Read the model definition and answer for the solid it produces. Units are mm, in the model's axes. A direction names the side the tool comes from. Round coordinates to 2 decimals unless told otherwise and drop trailing zeros. Order: outer loops, then holes, each group sorted by start corner. A loop starts at its lowest first (then second) coordinate and runs counter-clockwise, first axis right, second up.
from build123d import *

# Parameters (mm, degrees)
CROQUIS1_W              = 64
CROQUIS1_H              = 64
SALIENTE_EXTRUIR1_DEPTH = 60
CROQUIS2_W              = 70
CROQUIS2_H              = 70
CROQUIS2_W_2            = 64
CROQUIS2_H_2            = 64
SALIENTE_EXTRUIR2_DEPTH = 64
CORTAR_EXTRUIR1_DEPTH   = 21
CROQUIS5_R              = 1.1
CORTAR_EXTRUIR2_DEPTH   = 10
CORTAR_EXTRUIR3_REACH   = 30
CROQUIS10_R             = 4.5
CROQUIS11_W             = 70
CROQUIS11_H             = 70
CORTAR_EXTRUIR4_DEPTH   = 30
CROQUIS12_W             = 23
CROQUIS12_H             = 12.2
CORTAR_EXTRUIR5_DEPTH   = 21
CORTAR_EXTRUIR6_REACH   = 30
CROQUIS13_R             = 4.5
CROQUIS14_R             = 1.1
CORTAR_EXTRUIR7_DEPTH   = 10
CROQUIS15_R             = 3.7
CORTAR_EXTRUIR8_DEPTH   = 10
CROQUIS16_W             = 64
CROQUIS16_H             = 64
CORTAR_EXTRUIR9_DEPTH   = 5
CROQUIS17_W             = 12.5
CROQUIS17_H             = 12.998685397
CORTAR_EXTRUIR10_DEPTH  = 5
CORTAR_EXTRUIR11_REACH  = 72
CROQUIS18_W             = 70
CROQUIS18_H             = 9
CROQUIS18_H_2           = 5.000169364
CORTAR_EXTRUIR13_DEPTH  = 5
CORTAR_EXTRUIR14_REACH  = 12
CROQUIS21_W             = 81.467019472
CROQUIS21_H             = 81.467019472
CORTAR_EXTRUIR16_REACH  = 5.001
CROQUIS23_W             = 3.1
CROQUIS23_H             = 12.5


with BuildPart() as part:
    # Croquis1 → Saliente-Extruir1 (new body)
    with BuildSketch(Plane(origin=(0, 0, 0), x_dir=(1, 0, 0), z_dir=(0, 1, 0))):
        Rectangle(CROQUIS1_W, CROQUIS1_H)
    extrude(amount=SALIENTE_EXTRUIR1_DEPTH)

    # Croquis2 → Saliente-Extruir2 (add)
    with BuildSketch(Plane(origin=(0, 0, 0), x_dir=(1, 0, 0), z_dir=(0, 1, 0))):
        Rectangle(CROQUIS2_W, CROQUIS2_H)
        Rectangle(CROQUIS2_W_2, CROQUIS2_H_2, mode=Mode.SUBTRACT)
    extrude(amount=SALIENTE_EXTRUIR2_DEPTH)

    # Croquis4 → Cortar-Extruir1 (cut)
    with BuildSketch(Plane(origin=(0, 60, 0), x_dir=(1, 0, 0), z_dir=(0, 1, 0))):
        Polygon((-7, 6), (-7, -6), (-7, -6.25), (16, -6.25), (16, -6), (16, 6), (16, 6.25), (-7, 6.25), align=None)
    extrude(amount=-CORTAR_EXTRUIR1_DEPTH, mode=Mode.SUBTRACT)

    # Croquis5 → Cortar-Extruir2 (cut)
    with BuildSketch(Plane(origin=(0, 60, 0), x_dir=(1, 0, 0), z_dir=(0, 1, 0))):
        with Locations((19, 0)):
            Circle(CROQUIS5_R)
        with Locations((-9, 0)):
            Circle(CROQUIS5_R)
    extrude(amount=-CORTAR_EXTRUIR2_DEPTH, mode=Mode.SUBTRACT)

    # Croquis10 → Cortar-Extruir3 (cut, up to next)
    with BuildSketch(Plane(origin=(-7, 0, 0), x_dir=(0, 0, -1), z_dir=(1, 0, 0)), mode=Mode.PRIVATE) as cortar_extruir3_sk1:
        with Locations((0, 44)):
            Circle(CROQUIS10_R)
    cortar_extruir3_tool1 = extrude(cortar_extruir3_sk1.sketch, amount=-CORTAR_EXTRUIR3_REACH, mode=Mode.PRIVATE) & part.part
    add(cortar_extruir3_tool1.solids().sort_by_distance((-7, 44, 0))[0], mode=Mode.SUBTRACT)

    # Croquis11 → Cortar-Extruir4 (cut)
    with BuildSketch(Plane.XZ):
        Rectangle(CROQUIS11_W, CROQUIS11_H)
    extrude(amount=-CORTAR_EXTRUIR4_DEPTH, mode=Mode.SUBTRACT)

    # Croquis12 → Cortar-Extruir5 (cut)
    with BuildSketch(Plane.XZ.offset(-30)):
        with Locations((4.5, 22.1)):
            Rectangle(CROQUIS12_W, CROQUIS12_H)
    extrude(amount=-CORTAR_EXTRUIR5_DEPTH, mode=Mode.SUBTRACT)

    # Croquis13 → Cortar-Extruir6 (cut, up to next)
    with BuildSketch(Plane(origin=(-7, 0, 0), x_dir=(0, 0, -1), z_dir=(1, 0, 0)), mode=Mode.PRIVATE) as cortar_extruir6_sk1:
        with Locations((-22.1, 46)):
            Circle(CROQUIS13_R)
    cortar_extruir6_tool1 = extrude(cortar_extruir6_sk1.sketch, amount=-CORTAR_EXTRUIR6_REACH, mode=Mode.PRIVATE) & part.part
    add(cortar_extruir6_tool1.solids().sort_by_distance((-7, 46, 22.1))[0], mode=Mode.SUBTRACT)

    # Croquis14 → Cortar-Extruir7 (cut)
    with BuildSketch(Plane.XZ.offset(-30)):
        with Locations((19, 22.1)):
            Circle(CROQUIS14_R)
        with Locations((-9, 22.1)):
            Circle(CROQUIS14_R)
    extrude(amount=-CORTAR_EXTRUIR7_DEPTH, mode=Mode.SUBTRACT)

    # Croquis15 → Cortar-Extruir8 (cut)
    with BuildSketch(Plane.XZ.offset(-30)):
        with Locations((0, -22.1)):
            Circle(CROQUIS15_R)
    extrude(amount=-CORTAR_EXTRUIR8_DEPTH, mode=Mode.SUBTRACT)

    # Croquis16 → Cortar-Extruir9 (cut)
    with BuildSketch(Plane(origin=(0, 60, 0), x_dir=(1, 0, 0), z_dir=(0, 1, 0))):
        Rectangle(CROQUIS16_W, CROQUIS16_H)
    extrude(amount=-CORTAR_EXTRUIR9_DEPTH, mode=Mode.SUBTRACT)

    # Croquis17 → Cortar-Extruir10 (cut)
    with BuildSketch(Plane(origin=(-7, 0, 0), x_dir=(0, 0, -1), z_dir=(1, 0, 0))):
        with Locations((0, 45.499342699)):
            Rectangle(CROQUIS17_W, CROQUIS17_H)
    extrude(amount=-CORTAR_EXTRUIR10_DEPTH, mode=Mode.SUBTRACT)

    # Croquis18 → Cortar-Extruir11 (cut, up to next)
    with BuildSketch(Plane(origin=(35, 0, 0), x_dir=(0, 0, -1), z_dir=(1, 0, 0)), mode=Mode.PRIVATE) as cortar_extruir11_sk1:
        with Locations((0, 59.5)):
            Rectangle(CROQUIS18_W, CROQUIS18_H)
    cortar_extruir11_tool1 = extrude(cortar_extruir11_sk1.sketch, amount=-CORTAR_EXTRUIR11_REACH, mode=Mode.PRIVATE) & part.part
    add(cortar_extruir11_tool1.solids().sort_by_distance((35, 59.5, 0))[0], mode=Mode.SUBTRACT)
    # Croquis18 → Cortar-Extruir11 (cut, up to next)
    with BuildSketch(Plane(origin=(35, 0, 0), x_dir=(0, 0, -1), z_dir=(1, 0, 0)), mode=Mode.PRIVATE) as cortar_extruir11_sk2:
        with Locations((0, 32.500084682)):
            Rectangle(CROQUIS18_W, CROQUIS18_H_2)
    cortar_extruir11_tool2 = extrude(cortar_extruir11_sk2.sketch, amount=-CORTAR_EXTRUIR11_REACH, mode=Mode.PRIVATE) & part.part
    add(cortar_extruir11_tool2.solids().sort_by_distance((35, 32.500085, 0))[0], mode=Mode.SUBTRACT)

    # Croquis19 → Cortar-Extruir13 (cut)
    with BuildSketch(Plane(origin=(-7, 0, 0), x_dir=(0, 0, -1), z_dir=(1, 0, 0))):
        Polygon((-16, 51), (-28.2, 51), (-28.2, 38.000169364), (-22.1, 38.000169364), (-16, 38.000169364), align=None)
    extrude(amount=-CORTAR_EXTRUIR13_DEPTH, mode=Mode.SUBTRACT)

    # Croquis21 → Cortar-Extruir14 (cut, up to next)
    with BuildSketch(Plane(origin=(0, 45.000169364, 0), x_dir=(-1, 0, 0), z_dir=(0, -1, 0)), mode=Mode.PRIVATE) as cortar_extruir14_sk1:
        with Locations((0.076423095, -0.764230952)):
            Rectangle(CROQUIS21_W, CROQUIS21_H)
    cortar_extruir14_tool1 = extrude(cortar_extruir14_sk1.sketch, amount=CORTAR_EXTRUIR14_REACH, mode=Mode.PRIVATE) & part.part
    add(cortar_extruir14_tool1.solids().sort_by_distance((-0.076423, 45.000169, 0.764231))[0], mode=Mode.SUBTRACT)

    # Croquis23 → Cortar-Extruir16 (cut, up to next)
    with BuildSketch(Plane.XZ.offset(-51.998685397), mode=Mode.PRIVATE) as cortar_extruir16_sk1:
        with Locations((-8.55, 0)):
            Rectangle(CROQUIS23_W, CROQUIS23_H)
    cortar_extruir16_tool1 = extrude(cortar_extruir16_sk1.sketch, amount=-CORTAR_EXTRUIR16_REACH, mode=Mode.PRIVATE) & part.part
    add(cortar_extruir16_tool1.solids().sort_by_distance((-8.55, 51.998685, 0))[0], mode=Mode.SUBTRACT)


solid = part.part
Q1. A cutting plane is placed at C-C, the plane y = 46. Give the vertices of the cut face in (x, z).
Outcome:
outline: (-35, -35) - (35, -35) - (35, 35) - (-35, 35) - (-35, 26.6) - (-12, 26.6) - (-12, 28.2) - (16, 28.2) - (16, 16) - (-12, 16) - (-12, 17.6) - (-35, 17.6) - (-35, 4.03) - (-12, 4.03) - (-12, 6.25) - (16, 6.25) - (16, -6.25) - (-12, -6.25) - (-12, -4.03) - (-35, -4.03) - close
Q2. A cutting plane is placed at D-D, the plane x = 19. Give the vertices of the cut face in (y, z).
Outcome:
outline: (45, -35) - (55, -35) - (55, -1.1) - (50, -1.1) - (50, 1.1) - (55, 1.1) - (55, 35) - (45, 35) - close
Q3. A cutting plane is placed at B-B, the plane z = 22.1. Give the vertices of the cut face in (x, y), plus the area to 3 significant figures.
Outcome:
outline: (-35, 50.5) - (-12, 50.5) - (-12, 51) - (16, 51) - (16, 45) - (35, 45) - (35, 55) - (-35, 55) - close
area: 405 mm2
Q4. For a pull along X with two mould halves and no side action, classify faces 1 (the face through (16, 50, 0)), 2 (the face through (2, 48, 28.2)), 3 (the face through (35, 50, 0)), 4 (the face through (0, 45, -8)) as released by +X, released by -X, zero draft, split by the parting line, or undercut.
Outcome:
face 1: undercut
face 2: undercut
face 3: released by +X
face 4: zero draft
Q5. Flat-ended cylindrical pins translate along their axes: pin 1 (10 mm diameter, centred on x = 1.5, z = 23, fed in from -Y); pin 2 (0.6 mm diameter, centred on x = -10.5, z = -2, fed in from -Y); pin 3 (2 mm diameter, centred on x = 19, z = 0, fed in from +Y). Find the tip coordinate at first contact, or state that the pin passes through.
Outcome:
pin 1: stops at y = 51
pin 2: stops at y = 52
pin 3: stops at y = 50
Q6. For faces 5 (the face through (-23.3, 50.5, 22)), 6 (the face through (-11, 51.999, 0)), 7 (the face through (17.9, 52.5, 0)), determine the directions among +Z, -Z, +X, -X, +Y, -Y from which every point of the face is accessible in a straight line to the end or side of a thin tool.
Outcome:
face 5: -X
face 6: -Y
face 7: +Y
Q7. A cutting plane is placed at A-A, the plane z = 0. Give the vertices of the cut face in (x, y).
Outcome:
outline: (-35, 48.5) - (-12, 48.5) - (-12, 52) - (-10.1, 52) - (-10.1, 55) - (-35, 55) - close; (16, 45) - (35, 45) - (35, 55) - (20.1, 55) - (20.1, 50) - (17.9, 50) - (17.9, 55) - (16, 55) - close
Q8. Straight lines are drawn through the part: probe 1 along X at (y, z) = (52.15, 0); probe 2 along Z at (x, y) = (19, 50.75); probe 3 along Z at (x, y) = (-7, 48.75). For each, find the intervals that lie inside material, in ascending order.
Outcome:
probe 1: x = -35 to -10.1, 16 to 17.9, 20.1 to 35
probe 2: z = -35 to -1.1, 1.1 to 35
probe 3: z = -35 to -6.25, 6.25 to 16, 28.2 to 35
